```python
from build123d import *

# Parameters (mm, degrees)
SKETCH_1_R          = 2
SKETCH_1_R_2        = 4.5
SKETCH_1_R_3        = 1.65
EXTRUDE_1_DEPTH     = 4
FILLET_1_R          = 4
CUT_EXTRUDE_1_DEPTH = 10
FILLET_2_R          = 2


with BuildPart() as part:
    # 草图1 → 凸台-拉伸1 (new body)
    # profile 1 of 3: a face of its own
    with BuildSketch(Plane.XY):
        Polygon((-35, 10), (-35, -10), (35, -10), (35, 10), (-13.142135624, 10), align=None)
        with Locations((-30, -5)):
            Circle(SKETCH_1_R, mode=Mode.SUBTRACT)
        with Locations((-10, -5)):
            Circle(SKETCH_1_R, mode=Mode.SUBTRACT)
        with Locations((-30, 5)):
            Circle(SKETCH_1_R, mode=Mode.SUBTRACT)
        with Locations((-10, 5)):
            Circle(SKETCH_1_R, mode=Mode.SUBTRACT)
        Circle(SKETCH_1_R_2, mode=Mode.SUBTRACT)
        with Locations((10, -5)):
            Circle(SKETCH_1_R, mode=Mode.SUBTRACT)
        with Locations((10, 5)):
            Circle(SKETCH_1_R, mode=Mode.SUBTRACT)
        with Locations((30, -5)):
            Circle(SKETCH_1_R, mode=Mode.SUBTRACT)
        with Locations((30, 5)):
            Circle(SKETCH_1_R, mode=Mode.SUBTRACT)
    # profile 2 of 3: a face of its own
    with BuildSketch(Plane.XY):
        Polygon((-13.142135624, 10), (35, 10), (50, 25), (50, 73.142135624), align=None)
        with Locations((13.125631329, 29.196699141)):
            Circle(SKETCH_1_R_3, mode=Mode.SUBTRACT)
        with Locations((20.196699141, 22.125631329)):
            Circle(SKETCH_1_R_3, mode=Mode.SUBTRACT)
        with Locations((37.874368671, 39.803300859)):
            Circle(SKETCH_1_R_3, mode=Mode.SUBTRACT)
        with Locations((30.803300859, 46.874368671)):
            Circle(SKETCH_1_R_3, mode=Mode.SUBTRACT)
    # profile 3 of 3: a face of its own
    with BuildSketch(Plane.XY):
        Polygon((50, 73.142135624), (50, 25), (70, 25), (70, 95), (50, 95), align=None)
        with Locations((55, 30)):
            Circle(SKETCH_1_R, mode=Mode.SUBTRACT)
        with Locations((65, 30)):
            Circle(SKETCH_1_R, mode=Mode.SUBTRACT)
        with Locations((55, 50)):
            Circle(SKETCH_1_R, mode=Mode.SUBTRACT)
        with Locations((65, 50)):
            Circle(SKETCH_1_R, mode=Mode.SUBTRACT)
        with Locations((60, 60)):
            Circle(SKETCH_1_R_2, mode=Mode.SUBTRACT)
        with Locations((55, 70)):
            Circle(SKETCH_1_R, mode=Mode.SUBTRACT)
        with Locations((65, 70)):
            Circle(SKETCH_1_R, mode=Mode.SUBTRACT)
        with Locations((55, 90)):
            Circle(SKETCH_1_R, mode=Mode.SUBTRACT)
        with Locations((65, 90)):
            Circle(SKETCH_1_R, mode=Mode.SUBTRACT)
    extrude(amount=EXTRUDE_1_DEPTH)

    # 圆角1
    fillet_1_edges = [part.edges().sort_by_distance(p)[0] for p in [
        (35, 10, 2),
        (35, -10, 2),
        (-35, -10, 2),
        (-35, 10, 2),
        (-13.142135624, 10, 2),
        (50, 73.142135624, 2),
        (50, 95, 2),
        (70, 95, 2),
        (70, 25, 2),
        (50, 25, 2),
    ]]
    fillet(fillet_1_edges, radius=FILLET_1_R)

    # 草图2 → 切除-拉伸1 (cut)
    with BuildSketch(Plane.XY.offset(4)):
        Polygon((-8.087572106, 15.054563517), (-3.844931419, 19.297204204), (1.81192283, 13.640349955), (-2.430717857, 9.397709268), align=None)
        Polygon((44.945436483, 68.087572106), (40.702795796, 63.844931419), (46.359650045, 58.18807717), (50.602290732, 62.430717857), align=None)
    extrude(amount=-CUT_EXTRUDE_1_DEPTH, mode=Mode.SUBTRACT)

    # 圆角2
    fillet_2_edges = [part.edges().sort_by_distance(p)[0] for p in [
        (-2.430717857, 9.397709268, 2),
        (-8.087572106, 15.054563517, 2),
        (-3.844931419, 19.297204204, 2),
        (1.81192283, 13.640349955, 2),
        (44.945436483, 68.087572106, 2),
        (50.602290732, 62.430717857, 2),
        (46.359650045, 58.18807717, 2),
        (40.702795796, 63.844931419, 2),
    ]]
    fillet(fillet_2_edges, radius=FILLET_2_R)


solid = part.part
```
The model under review builds one solid part; all positions refer to its coordinate system, in mm. A direction names the side the tool comes from. Round coordinates to 2 decimals unless told otherwise and drop trailing zeros. Loops run counter-clockwise (first coordinate to the right, second up) from the corner with the lowest first, then second, coordinate; pieces in that order, holes last. Notation, with made-up numbers: (47, -34) - (102, -34) arc R25 ccw to (102, 1) - close; hole circle Ø4 at (56.25, -24). An arc over 180 degrees is marked (long way). Write each question's results on one line, items separated by ' | '. Start each with the question number.
Q1. Take a section at A-A on y = 0. Give the boundary of the cut face in (x, z), plus the area to 3 significant figures.
Q2. Draft analysis for pull direction X (two halves, no side actions). For faces 1 (the cylindrical face through (-11.6, -6.2, 2)), 2 (the flat face through (35, 1, 2)), 3 (the cylindrical face through (-3.016, 19.275, 1.972)), state which applies: pulls with the +X half, pulls with the -X half, needs draft (parallel to the pull), parting line crosses it, or undercut.
Q3. Take a section at C-C on z = 2. Give the number of separate pieces and of enclosed holes in the cut face, plus the area to 3 significant figures.
Q4. Insertion check: P1, Ø1.2, axis at y = 82, z = 1, coming from the -X side; P2, Ø3, axis at x = -30, y = -5, coming from the -Z side; P3, Ø1.2, axis at x = -24.5, z = 3, coming from the +Y side. Each pin has a flat end and moves straight along its axis. Give the tip position at first contact, or say it passes through.
Q5. Take a section at D-D on y = 33.5. Give the boundary of the cut face in (x, z).
Q6. Wall thickness on line 1 along Y through (x, z) = (65, 0.9); line 2 along Y through (x, z) = (-30, 3.45); line 3 along Y through (x, z) = (0, 3.7): over which ranges is each line inside the solid? List them lowest first. Write a range as [from, to].
Q7. Tool access review of faces 4 (the cylindrical face through (49.774, 62.409, 1.972)), 5 (the flat face through (50, 83, 2)), 6 (the flat face through (-1.04, 16.49, 2.03)): name each direction out of +Z, -Z, +X, -X, +Y, -Y from which nothing blocks a thin tool from reaching the whole face with its end or side.
Q8. Take a section at B-B on y = 50. Give the boundary of the cut face in (x, z).
Data:
1) outline: (-35, 0) - (-4.5, 0) - (-4.5, 4) - (-35, 4) - close; (4.5, 0) - (35, 0) - (35, 4) - (4.5, 4) - close | area: 244 mm²
2) face 1: undercut | face 2: pulls with the +X half | face 3: pulls with the -X half
3) separate pieces: 1 | enclosed holes: 22 | area: 4,200 mm²
4) P1: stops at x = 50 | P2: passes through | P3: stops at y = 10
5) outline: (10.36, 0) - (70, 0) - (70, 4) - (10.36, 4) - close
6) line 1: y = [25, 28], [32, 48], [52, 68], [72, 88], [92, 95] | line 2: y = [-10, -7], [-3, 3], [7, 10] | line 3: y = [-10, -4.5], [4.5, 11.83], [15.45, 23.14]
7) face 4: +Z, -Z | face 5: +Z, -Z, -X, +Y | face 6: +Z, -Z, -X
8) outline: (26.86, 0) - (53, 0) - (53, 4) - (26.86, 4) - close; (57, 0) - (63, 0) - (63, 4) - (57, 4) - close; (67, 0) - (70, 0) - (70, 4) - (67, 4) - close
